Answer from the drawing. Dimensions are ordinates in mm from the lowest x, y and z of the part. A direction names the side the tool comes from. Round coordinates to 2 decimals unless told otherwise and drop trailing zeros. Return JSON: item names as keys, results as strings. Group by question number.
(1) Straight lines are drawn through the part: line 1 (X direction, y = 2.25, z = 2.9); line 2 (Y direction, x = 12.5, z = 2.55); line 3 (Y direction, x = 1.75, z = 0.6) (1 decimal). For each, find the intervals that lie inside material, in ascending order.
(2) For the marked faces 5 and 6, determine the directions among +Z, -Z, +X, -X, +Y, -Y from which every point of the face is accessible in a straight line to the end or side of a thin tool.
(3) A cutting plane is placed at C-C on z = 0.75. State how many separate pieces and enclosed holes the cut face has, then the cut area to 3 significant figures.
(4) The mould has two halves that part along X. Classify the marked faces 1, 2, 3 and 4: released by +X, released by -X, zero draft, split by the parting line, or undercut.
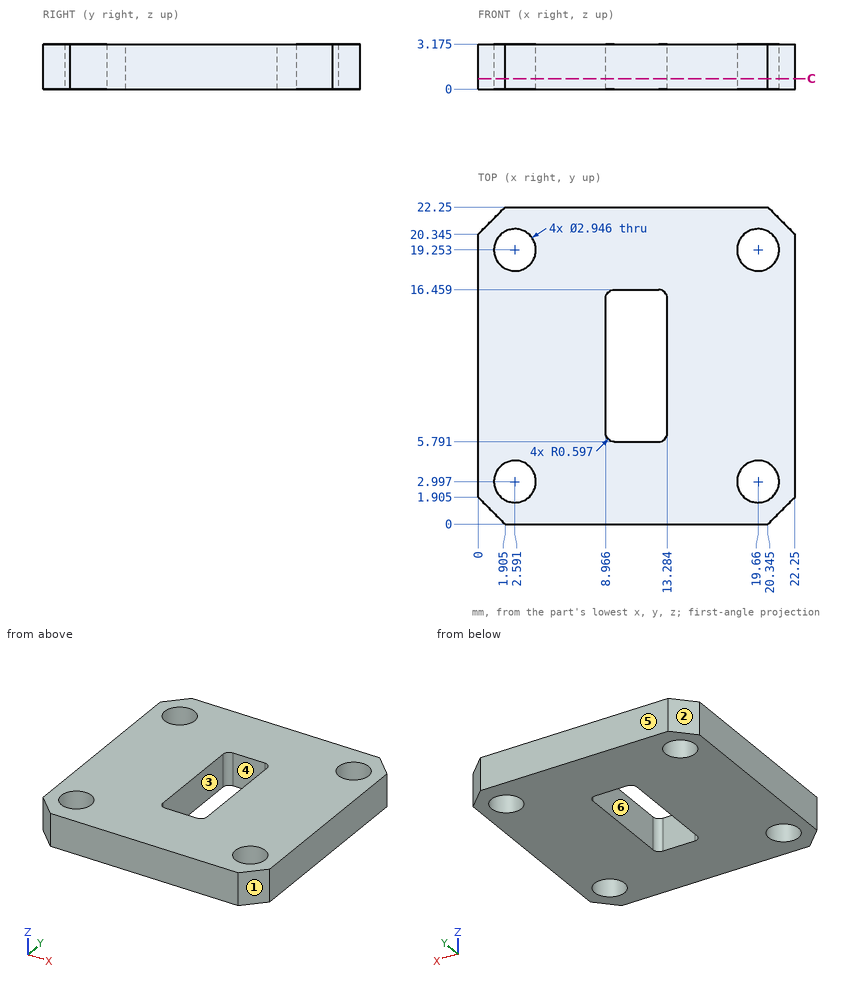
Checks:
{
 "1": {"line 1": "x = 0 to 1.32, 3.86 to 18.39, 20.93 to 22.25", "line 2": "y = 0 to 5.79, 16.46 to 22.25", "line 3": "y = 0.2 to 1.8, 4.2 to 18, 20.5 to 22.1"},
 "2": {"face 5": "+Z, -Z, +X, -X, +Y", "face 6": "+Z, -Z"},
 "3": {"separate pieces": "1", "enclosed holes": "5", "area": "415 mm^2"},
 "4": {"face 1": "released by +X", "face 2": "released by -X", "face 3": "undercut", "face 4": "undercut"}
}
